Work out the finished part from the listing and answer in its coordinate system (mm). A direction names the side the tool comes from. Give positions to 0.01 mm unless a question says otherwise; leave off trailing zeros. Loops run counter-clockwise (first coordinate to the right, second up) from the corner with the lowest first, then second, coordinate; pieces in that order, holes last.
```python
from build123d import *

# Parameters (mm, degrees)
BOX003_W         = 10
BOX003_H         = 110
BOX003_DEPTH     = 10
ARRAY001_X_COUNT = 4
ARRAY001_X_PITCH = 20
BOX002_W         = 110
BOX002_H         = 10
BOX002_DEPTH     = 10
ARRAY_X_COUNT    = 4
ARRAY_X_PITCH    = 20
BOX001_W         = 70
BOX001_H         = 70
BOX001_DEPTH     = 70
BOX_W            = 90
BOX_H            = 90
BOX_DEPTH        = 150


with BuildPart() as fusion001:
    # Box003 → Box003 (new body)
    with BuildSketch(Plane(origin=(10, -10, 140), x_dir=(1, 0, 0), z_dir=(0, 0, 1))):
        with Locations((5, 55)):
            Rectangle(BOX003_W, BOX003_H)
    extrude(amount=BOX003_DEPTH)

    # Array001 X: Fusion001 ×4


with BuildPart() as fusion001_1:
    add(fusion001.part)
    with Locations(*[(i * ARRAY001_X_PITCH, 0, 0) for i in range(1, ARRAY001_X_COUNT)]):
        add(fusion001.part)


with BuildPart() as fusion002:
    # Box002 → Box002 (new body)
    with BuildSketch(Plane(origin=(-10, 10, 140), x_dir=(1, 0, 0), z_dir=(0, 0, 1))):
        with Locations((55, 5)):
            Rectangle(BOX002_W, BOX002_H)
    extrude(amount=BOX002_DEPTH)

    # Array X: Fusion002 ×4


with BuildPart() as fusion002_1:
    add(fusion002.part)
    with Locations(*[(0, i * ARRAY_X_PITCH, 0) for i in range(1, ARRAY_X_COUNT)]):
        add(fusion002.part)

    # Fusion002: union Fusion001
    add(fusion001_1.part)


with BuildPart() as cube001:
    # Box001 → Box001 (new body)
    with BuildSketch(Plane(origin=(10, 10, 115), x_dir=(1, 0, 0), z_dir=(0, 0, 1))):
        with Locations((35, 35)):
            Rectangle(BOX001_W, BOX001_H)
    extrude(amount=BOX001_DEPTH)


with BuildPart() as torre:
    # Box → Box (new body)
    with BuildSketch(Plane.XY):
        with Locations((45, 45)):
            Rectangle(BOX_W, BOX_H)
    extrude(amount=BOX_DEPTH)

    # Cut: cut Cube001
    add(cube001.part, mode=Mode.SUBTRACT)

    # Cut001: cut Fusion002
    add(fusion002_1.part, mode=Mode.SUBTRACT)


solid = torre.part
```
Q1. Consider line 1 along Y through (x, z) = (36.5, 134.5); line 2 along Z through (x, y) = (36, 61). Determine where each line is inside the solid, lowest interval first.
Q2. Determine the mould class of faces 1 (the face through (35, 5, 140)), 2 (the face through (65, 5, 150)), 3 (the face through (30, 85, 145)) for opening direction X: +X half, -X half, draft (parallel to the pull), parting line (faces both ways), or undercut.
Q3. Which of the six approach directions +Z, -Z, +X, -X, +Y, -Y give full straight-line access (tool end or side, diameter ignored) to faces 4 (the face through (85, 45, 150)), 5 (the face through (80, 45, 128)), 6 (the face through (85, 60, 145)), 7 (the face through (15, 85, 140))?
Q4. Section C-C on y = 83 is taken. Give the vertices of the cut face in (x, z), plus the area to 3 significant figures.
Q5. Section B-B on z = 125 is taken. Give the vertices of the cut face in (x, y), plus the area to 3 significant figures.
Q6. Given pin 1 (5 mm diameter, centred on x = 34.5, y = 84.5, fed in from +Z); pin 2 (2 mm diameter, centred on x = 32, y = 59, fed in from +Z), each flat-ended and moving along its own axis, determine where each tip first touches the part or whether it passes through.
Q7. Section D-D on x = 68 is taken. Give the vertices of the cut face in (y, z), plus the area to 4 significant figures.
Q8. Section A-A on x = 14 is taken. Give the vertices of the cut face in (y, z), plus the area to 4 significant figures.
Check result:
1. line 1: y = 0 to 10, 80 to 90
1. line 2: z = 0 to 115
2. face 1: undercut
2. face 2: draft
2. face 3: undercut
3. face 4: +Z, +X, -X, +Y, -Y
3. face 5: +Z
3. face 6: +Z, +X, -X
3. face 7: +Z, +Y, -Y
4. outline: (0, 0) - (90, 0) - (90, 150) - (80, 150) - (80, 140) - (70, 140) - (70, 150) - (60, 150) - (60, 140) - (50, 140) - (50, 150) - (40, 150) - (40, 140) - (30, 140) - (30, 150) - (20, 150) - (20, 140) - (10, 140) - (10, 150) - (0, 150) - close
4. area: 13,100 mm2
5. outline: (0, 0) - (90, 0) - (90, 90) - (0, 90) - close; hole (10, 10) - (80, 10) - (80, 80) - (10, 80) - close
5. area: 3,200 mm2
6. pin 1: stops at z = 140
6. pin 2: stops at z = 115
7. outline: (0, 0) - (90, 0) - (90, 150) - (80, 150) - (80, 115) - (10, 115) - (10, 150) - (0, 150) - close
7. area: 11,050 mm2
8. outline: (0, 0) - (90, 0) - (90, 140) - (80, 140) - (80, 115) - (10, 115) - (10, 140) - (0, 140) - close
8. area: 10,850 mm2
